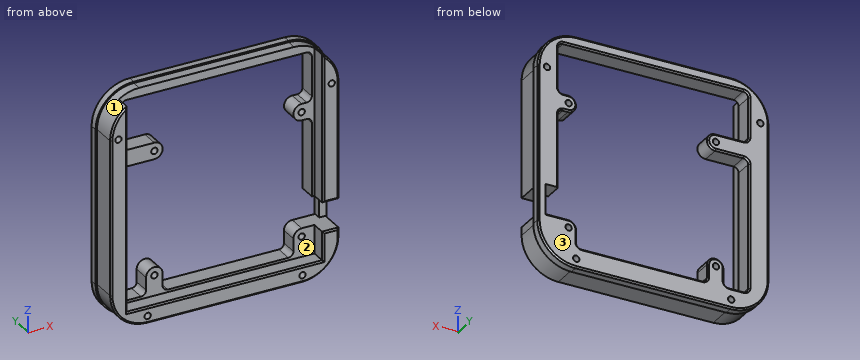
```python
from build123d import *

# Parameters (mm, degrees)
SKETCH1_W                   = 91
SKETCH1_H                   = 91
SKETCH1_R                   = 1.25
BOSS_EXTRUDE1_DEPTH         = 7.4
SKETCH3_W                   = 5
SKETCH3_H                   = 11.5
CUT_EXTRUDE1_DEPTH          = 8.4
SKETCH4_W                   = 91
SKETCH4_H                   = 91
BOSS_EXTRUDE2_DEPTH         = 6.1
FILLET1_R                   = 15
CUT_EXTRUDE2_DEPTH          = 10
SKETCH9_W                   = 11.5
SKETCH9_H                   = 10
CUT_EXTRUDE3_DEPTH          = 10
CUT_EXTRUDE4_DEPTH          = 6.1
FILLET2_R                   = 2
TAP_DRILL_FOR_M3X0_5_TAP1_D = 2.5
CHAMFER1_SIZE               = 0.6


with BuildPart() as part:
    # Sketch1 → Boss-Extrude1 (new body)
    with BuildSketch(Plane(origin=(0, 0, 0), x_dir=(1, 0, 0), z_dir=(0, 1, 0))):
        with Locations((-1.280392157, -3.837254902)):
            Rectangle(SKETCH1_W, SKETCH1_H)
        with BuildLine():
            Line((28.969607843, 33.662745098), (28.969607843, 26.662745098))
            ThreePointArc((28.969607843, 26.662745098), (29.921510804, 24.364648059), (32.219607843, 23.412745098))
            Line((32.219607843, 23.412745098), (36.219607843, 23.412745098))
            Line((36.219607843, 23.412745098), (36.219607843, -19.087254902))
            Line((36.219607843, -19.087254902), (32.219607843, -19.087254902))
            ThreePointArc((32.219607843, -19.087254902), (28.969607843, -22.337254902), (32.219607843, -25.587254902))
            Line((32.219607843, -25.587254902), (36.219607843, -25.587254902))
            Line((36.219607843, -25.587254902), (36.219607843, -45.337254902))
            Line((36.219607843, -45.337254902), (-38.780392157, -45.337254902))
            Line((-38.780392157, -45.337254902), (-38.780392157, -25.587254902))
            Line((-38.780392157, -25.587254902), (-25.780392157, -25.587254902))
            ThreePointArc((-25.780392157, -25.587254902), (-22.530392157, -22.337254902), (-25.780392157, -19.087254902))
            Line((-25.780392157, -19.087254902), (-38.780392157, -19.087254902))
            Line((-38.780392157, -19.087254902), (-38.780392157, 33.662745098))
            Line((-38.780392157, 33.662745098), (-29.030392157, 33.662745098))
            Line((-29.030392157, 33.662745098), (-29.030392157, 26.662745098))
            ThreePointArc((-29.030392157, 26.662745098), (-25.780392157, 23.412745098), (-22.530392157, 26.662745098))
            Line((-22.530392157, 26.662745098), (-22.530392157, 33.662745098))
            Line((-22.530392157, 33.662745098), (28.969607843, 33.662745098))
        make_face(mode=Mode.SUBTRACT)
        with Locations((32.219607843, 26.662745098)):
            Circle(SKETCH1_R, mode=Mode.SUBTRACT)
        with Locations((-25.780392157, 26.662745098)):
            Circle(SKETCH1_R, mode=Mode.SUBTRACT)
        with Locations((32.219607843, -22.337254902)):
            Circle(SKETCH1_R, mode=Mode.SUBTRACT)
        with Locations((-25.780392157, -22.337254902)):
            Circle(SKETCH1_R, mode=Mode.SUBTRACT)
    extrude(amount=BOSS_EXTRUDE1_DEPTH)

    # Sketch3 → Cut-Extrude1 (cut, through all)
    with BuildSketch(Plane.XZ):
        with Locations((38.719607843, -17.662745098)):
            Rectangle(SKETCH3_W, SKETCH3_H)
    extrude(amount=-CUT_EXTRUDE1_DEPTH, mode=Mode.SUBTRACT)

    # Sketch4 → Boss-Extrude2 (add)
    with BuildSketch(Plane.XZ):
        with Locations((-1.280392157, 3.837254902)):
            Rectangle(SKETCH4_W, SKETCH4_H)
        Polygon((37.219607843, 45.337254902), (37.219607843, -11.912745098), (41.219607843, -11.912745098), (41.219607843, -23.412745098), (37.219607843, -23.412745098), (37.219607843, -33.662745098), (37.219607843, -34.662745098), (36.219607843, -34.662745098), (-39.780392157, -34.662745098), (-39.780392157, 25.587254902), (-39.780392157, 45.337254902), (-39.780392157, 46.337254902), (-38.780392157, 46.337254902), (36.219607843, 46.337254902), (37.219607843, 46.337254902), align=None, mode=Mode.SUBTRACT)
    extrude(amount=BOSS_EXTRUDE2_DEPTH)

    # Fillet1
    fillet1_edges = [part.edges().sort_by_distance(p)[0] for p in [
        (-46.780392157, 0.65, 49.337254902),
        (-46.780392157, 0.65, -41.662745098),
        (44.219607843, 0.65, -41.662745098),
        (44.219607843, 0.65, 49.337254902),
    ]]
    fillet(fillet1_edges, radius=FILLET1_R)

    # Sketch8 → Cut-Extrude2 (cut)
    with BuildSketch(Plane.XZ.offset(6.1)):
        with BuildLine():
            Line((29.219607843, 49.337254902), (-31.780392157, 49.337254902))
            ThreePointArc((-31.780392157, 49.337254902), (-42.386993875, 44.94385662), (-46.780392157, 34.337254902))
            Line((-46.780392157, 34.337254902), (-46.780392157, -26.662745098))
            ThreePointArc((-46.780392157, -26.662745098), (-42.386993875, -37.269346816), (-31.780392157, -41.662745098))
            Line((-31.780392157, -41.662745098), (29.219607843, -41.662745098))
            ThreePointArc((29.219607843, -41.662745098), (39.826209561, -37.269346816), (44.219607843, -26.662745098))
            Line((44.219607843, -26.662745098), (44.219607843, 34.337254902))
            ThreePointArc((44.219607843, 34.337254902), (39.826209561, 44.94385662), (29.219607843, 49.337254902))
        make_face()
        with BuildLine():
            Line((29.219607843, 48.787254902), (-31.780392157, 48.787254902))
            ThreePointArc((-31.780392157, 48.787254902), (-41.998085145, 44.55494789), (-46.230392157, 34.337254902))
            Line((-46.230392157, 34.337254902), (-46.230392157, -26.662745098))
            ThreePointArc((-46.230392157, -26.662745098), (-41.998085145, -36.880438086), (-31.780392157, -41.112745098))
            Line((-31.780392157, -41.112745098), (29.219607843, -41.112745098))
            ThreePointArc((29.219607843, -41.112745098), (39.437300831, -36.880438086), (43.669607843, -26.662745098))
            Line((43.669607843, -26.662745098), (43.669607843, 34.337254902))
            ThreePointArc((43.669607843, 34.337254902), (39.437300831, 44.55494789), (29.219607843, 48.787254902))
        make_face(mode=Mode.SUBTRACT)
    extrude(amount=-CUT_EXTRUDE2_DEPTH, mode=Mode.SUBTRACT)

    # Sketch9 → Cut-Extrude3 (cut)
    with BuildSketch(Plane(origin=(43.669607843, 0, 0), x_dir=(0, 0, -1), z_dir=(1, 0, 0))):
        with Locations((17.662745098, -1.1)):
            Rectangle(SKETCH9_W, SKETCH9_H)
    extrude(amount=-CUT_EXTRUDE3_DEPTH, mode=Mode.SUBTRACT)

    # Sketch10 → Cut-Extrude4 (cut)
    with BuildSketch(Plane.XZ.offset(6.1)):
        with BuildLine():
            Line((-39.780392157, 46.337254902), (37.219607843, 46.337254902))
            Line((37.219607843, 46.337254902), (37.219607843, 46.370645945))
            ThreePointArc((37.219607843, 46.370645945), (33.398124292, 48.169915539), (29.219607843, 48.787254902))
            Line((29.219607843, 48.787254902), (-31.780392157, 48.787254902))
            ThreePointArc((-31.780392157, 48.787254902), (-35.958908606, 48.169915539), (-39.780392157, 46.370645945))
            Line((-39.780392157, 46.370645945), (-39.780392157, 46.337254902))
        make_face()
    extrude(amount=-CUT_EXTRUDE4_DEPTH, mode=Mode.SUBTRACT)

    # Fillet2
    fillet2_edges = [part.edges().sort_by_distance(p)[0] for p in [
        (-29.030392157, 3.7, -33.662745098),
        (-38.780392157, 3.7, -33.662745098),
        (-38.780392157, 3.7, 19.087254902),
        (-38.780392157, 3.7, 25.587254902),
        (-38.780392157, 3.7, 45.337254902),
        (36.219607843, 3.7, 45.337254902),
        (36.219607843, 3.7, 25.587254902),
        (36.219607843, 3.7, 19.087254902),
        (28.969607843, 3.7, -33.662745098),
        (-22.530392157, 3.7, -33.662745098),
    ]]
    fillet(fillet2_edges, radius=FILLET2_R)

    # Tap Drill for M3x0.5 Tap1 (through all)
    with Locations(Plane(origin=(-31.780392157, 7.4, -38.162745098), x_dir=(0, 0, 1), z_dir=(0, 1, 0))):
        with Locations((0, 0), (0, 61), (72.5, -11.5), (72.5, 72.5)):
            Hole(TAP_DRILL_FOR_M3X0_5_TAP1_D / 2)

    # Chamfer1
    chamfer1_edges = [part.edges().sort_by_distance(p)[0] for p in [
        (-29.030392157, 7.4, -29.162745098),
        (37.219607843, -6.1, 17.228950424),
        (37.219607843, -6.1, -29.037745098),
        (40.444607843, -6.1, -11.912745098),
        (40.444607843, -6.1, -23.412745098),
        (-1.280392157, -6.1, -34.662745098),
        (-39.780392157, -6.1, 5.853950424),
        (-1.280392157, 7.4, 49.337254902),
        (-46.780392157, 7.4, 3.837254902),
        (44.219607843, 7.4, 3.837254902),
        (-1.280392157, 7.4, -41.662745098),
        (-42.386993875, 7.4, -37.269346816),
        (39.826209561, 7.4, -37.269346816),
        (39.826209561, 7.4, 44.94385662),
        (-42.386993875, 7.4, 44.94385662),
        (-25.780392157, 7.4, -23.412745098),
        (41.955433297, -6.1, 41.163765724),
        (43.669607843, -6.1, -25.037745098),
        (39.437300831, -6.1, -36.880438086),
        (-1.280392157, -6.1, -41.112745098),
        (-41.998085145, -6.1, -36.880438086),
        (-46.230392157, -6.1, 3.837254902),
        (-22.530392157, 7.4, -29.162745098),
        (43.669607843, -6.1, 11.212254902),
        (-44.516217611, -6.1, 41.163765724),
        (-38.780392157, 7.4, -7.287745098),
        (-38.780392157, 7.4, 35.462254902),
        (36.219607843, 7.4, 35.462254902),
        (-33.905392157, 7.4, -33.662745098),
        (3.219607843, 7.4, -33.662745098),
        (-1.280392157, 7.4, 45.337254902),
        (-38.194605719, 7.4, 18.501468464),
        (-38.194605719, 7.4, 26.17304134),
        (35.633821406, 7.4, 26.17304134),
        (28.969607843, 7.4, -29.162745098),
        (35.633821406, 7.4, 18.501468464),
        (-38.194605719, 7.4, -33.07695866),
        (-29.616178594, 7.4, -33.07695866),
        (-21.944605719, 7.4, -33.07695866),
        (28.383821406, 7.4, -33.07695866),
        (-38.194605719, 7.4, 44.751468464),
        (35.633821406, 7.4, 44.751468464),
        (29.921510804, 7.4, -24.364648059),
        (36.719607843, 7.4, -23.412745098),
        (33.219607843, 7.4, 19.087254902),
        (28.969607843, 7.4, 22.337254902),
        (33.219607843, 7.4, 25.587254902),
        (-31.280392157, 7.4, 25.587254902),
        (-22.530392157, 7.4, 22.337254902),
        (36.219607843, 7.4, 2.587254902),
        (-31.280392157, 7.4, 19.087254902),
    ]]
    chamfer(chamfer1_edges, length=CHAMFER1_SIZE)


solid = part.part
```
Build history of the part. All positions in model axes, mm. Face numbers are marked on the shaded views. A direction names the side the tool comes from. Coordinates: 2 decimals unless noted, no trailing zeros. Order: outer loops, then holes, each group sorted by start corner. A loop starts at its lowest first (then second) coordinate and runs counter-clockwise, first axis right, second up. Notation, with made-up numbers: (-16.5, 30.5) -> (7.5, 30.5) arc R25 ccw to (7.5, 52.5) -> close; hole circle Ø8 at (87, 55). An arc over 180 degrees is marked (long way). Answer in a Markdown table with one row per item. Add a question column.
Q1. Band-saw the part on B-B, the plane z = 11. List the corners of the cut face in (x, y).
Q2. Band-saw the part on D-D, the plane z = -13. List the corners of the cut face in (x, y), then the cut area to 3 significant figures.
Q3. Wall check: line 1 along X through (y, z) = (2.5, 16); line 2 along Z through (x, y) = (-14.5, 1.5); line 3 along X through (y, z) = (6, 30.5). Give the ranges that are in metal, low to high. Write a range as [from, to].
Q4. Which spindle directions (+Z, -Z, +X, -X, +Y, -Y) get a long thin tool onto all of the face, cutting with end or side? Do the marked faces 1, 2 and 3. Say none if no direction does.
Q5. Drop flat-ended pins along their axis: pin 1 (3 mm diameter, centred on y = -2.5, z = 23, fed in from -X); pin 2 (8 mm diameter, centred on x = 25.5, y = -2.5, fed in from -Z); pin 3 (2 mm diameter, centred on x = 40.72, z = 34.34, fed in from +Y); pin 4 (12 mm diameter, centred on x = -19, z = -28.5, fed in from +Y). Give the stop position or say it passes through.
Q6. Band-saw the part on C-C, the plane y = -1.25. List the corners of the cut face in (x, z).
Q7. Band-saw the part on A-A, the plane x = -11. List the corners of the cut face in (y, z).
Answers follow:
| question | item | result |
|---|---|---|
| 1 | outline | (-46.78, 3.9) -> (-46.23, 3.9) -> (-46.23, -5.5) -> (-45.63, -6.1) -> (-40.38, -6.1) -> (-39.78, -5.5) -> (-39.78, 0) -> (-38.78, 0) -> (-38.78, 6.8) -> (-39.38, 7.4) -> (-46.18, 7.4) -> (-46.78, 6.8) -> close; (36.22, 0) -> (37.22, 0) -> (37.22, -5.5) -> (37.82, -6.1) -> (43.07, -6.1) -> (43.67, -5.5) -> (43.67, 3.9) -> (44.22, 3.9) -> (44.22, 6.8) -> (43.62, 7.4) -> (36.82, 7.4) -> (36.22, 6.8) -> close |
| 2 | outline | (-46.78, 3.9) -> (-46.23, 3.9) -> (-46.23, -5.5) -> (-45.63, -6.1) -> (-40.38, -6.1) -> (-39.78, -5.5) -> (-39.78, 0) -> (-38.78, 0) -> (-38.78, 6.8) -> (-39.38, 7.4) -> (-46.18, 7.4) -> (-46.78, 6.8) -> close; (41.22, 3.9) -> (44.22, 3.9) -> (44.22, 6.8) -> (43.62, 7.4) -> (41.22, 7.4) -> close |
| 2 | area | 106 mm^2 |
| 3 | line 1 | [-46.23, -38.78], [36.22, 43.67] |
| 3 | line 2 | [-41.11, -33.66], [45.34, 48.79] |
| 3 | line 3 | [-46.78, -38.78], [36.22, 44.22] |
| 4 | face 1 | +Z, -X, -Y |
| 4 | face 2 | +Z, -Y |
| 4 | face 3 | +Z, -Z, +X, -X, +Y |
| 5 | pin 1 | x = -46.23 |
| 5 | pin 2 | z = -41.11 |
| 5 | pin 3 | through |
| 5 | pin 4 | y = 7.4 |
| 6 | outline | (-46.23, -26.66) arc R14.45 ccw to (-31.78, -41.11) -> (29.22, -41.11) arc R14.45 ccw to (43.67, -26.66) -> (43.67, -23.41) -> (37.22, -23.41) -> (37.22, -34.66) -> (-39.78, -34.66) -> (-39.78, 46.37) arc R14.45 ccw to (-46.23, 34.34) -> close; (37.22, -11.91) -> (43.67, -11.91) -> (43.67, 34.34) arc R14.45 ccw to (37.22, 46.37) -> close; hole circle Ø2.5 at (-43.28, 34.34); hole circle Ø2.5 at (-31.78, -38.16); hole circle Ø2.5 at (29.22, -38.16); hole circle Ø2.5 at (40.72, 34.34) |
| 7 | outline | (-6.1, -40.51) -> (-5.5, -41.11) -> (3.9, -41.11) -> (3.9, -41.66) -> (6.8, -41.66) -> (7.4, -41.06) -> (7.4, -34.26) -> (6.8, -33.66) -> (0, -33.66) -> (0, -34.66) -> (-5.5, -34.66) -> (-6.1, -35.26) -> close; (0, 45.34) -> (6.8, 45.34) -> (7.4, 45.94) -> (7.4, 48.74) -> (6.8, 49.34) -> (3.9, 49.34) -> (3.9, 48.79) -> (0, 48.79) -> close |
